from build123d import *

# Parameters (mm, degrees)
SKETCH046_R           = 18.65
SKETCH046_R_2         = 6.05
PAD013_DEPTH          = 2
HOLE001_D             = 3
HOLE001_CSINK_D       = 6.1
HOLE001_CSINK_ANGLE   = 90
POLARPATTERN002_COUNT = 5


with BuildPart() as part:
    # Sketch046 → Pad013 (new body)
    with BuildSketch(Plane.XY.offset(20.5)):
        Circle(SKETCH046_R)
        Circle(SKETCH046_R_2, mode=Mode.SUBTRACT)
    extrude(amount=PAD013_DEPTH)

    # Hole001 (through all)
    with Locations(Plane.XY.offset(22.5)):
        with Locations((10.881279, 7.905712)):
            hole001 = CounterSinkHole(HOLE001_D / 2, HOLE001_CSINK_D / 2, counter_sink_angle=HOLE001_CSINK_ANGLE)

    # PolarPattern002: Hole001 ×5 about axis
    polarpattern002_axis = Axis((0, 0, 22.5), (0, 0, 1))
    for i in range(1, POLARPATTERN002_COUNT):
        add(hole001.rotate(polarpattern002_axis, i * 360 / POLARPATTERN002_COUNT), mode=Mode.SUBTRACT)


solid = part.part
The model under review builds one solid part; all positions refer to its coordinate system, in mm. Give positions to 0.01 mm unless a question says otherwise; leave off trailing zeros. Loops run counter-clockwise (first coordinate to the right, second up) from the corner with the lowest first, then second, coordinate; pieces in that order, holes last. Notation, with made-up numbers: (77, 6) -> (86, 6) arc R18 cw to (86, 29) -> close; hole circle Ø5 at (-11.75, 22.5). An arc over 180 degrees is marked (long way). Answer as a JSON object with one key per item and string values. Group by question number.
Q1. Take a section at D-D (x = 4.5). Write out the cut boundary in (y, z), plus the area to 3 significant figures.
Q2. Wall thickness on line 1 along Y through (x, z) = (0, 21); line 2 along Y through (x, z) = (13, 21.9); line 3 along X through (y, z) = (-2, 21.75): over which ranges is each line inside the solid? List them lowest first.
Q3. Take a section at C-C (z = 22.1). Write out the cut boundary in (x, y).
Q4. Take a section at B-B (x = 0). Write out the cut boundary in (y, z).
Q5. Insertion check: pin 1 (1.8 mm diameter, centred on x = -4.16, y = -12.79, fed in from +Z); pin 2 (4 mm diameter, centred on x = 10.88, y = -7.91, fed in from +Z); pin 3 (1 mm diameter, centred on x = 14, z = 21.5, fed in from +Y). Each pin has a flat end and moves straight along its axis. Give the tip position at first contact, or say it passes through.
Q6. Take a section at A-A (y = 0). Write out the cut boundary in (x, z).
Q7. Draft analysis for pull direction Y (two halves, no side actions). For faces 1 (the cylindrical face through (9.59, -8.67, 20.72)), 2 (the cylindrical face through (-14.8, -11.35, 21.49)), 3 (the flat face through (-4.4, 4.4, 20.5)), state which applies: pulls with the +Y half, pulls with the -Y half, needs draft (parallel to the pull), parting line crosses it, or undercut.
Answer below:
{
 "1": {"outline": "(-18.1, 20.5) -> (-4.04, 20.5) -> (-4.04, 22.5) -> (-18.1, 22.5) -> close; (4.04, 20.5) -> (18.1, 20.5) -> (18.1, 22.5) -> (4.04, 22.5) -> close", "area": "56.2 mm2"},
 "2": {"line 1": "y = -18.65 to -6.05, 6.05 to 18.65", "line 2": "y = -13.37 to -9.14, -6.68 to 6.68, 9.14 to 13.37", "line 3": "x = -18.54 to -14.59, -12.31 to -5.71, 5.71 to 18.54"},
 "3": {"outline": "circle Ø37.3 at (0, 0); hole circle Ø5.3 at (-13.45, 0); hole circle Ø5.3 at (-4.16, -12.79); hole circle Ø5.3 at (-4.16, 12.79); hole circle Ø12.1 at (0, 0); hole circle Ø5.3 at (10.88, -7.91); hole circle Ø5.3 at (10.88, 7.91)"},
 "4": {"outline": "(-18.65, 20.5) -> (-6.05, 20.5) -> (-6.05, 22.5) -> (-18.65, 22.5) -> close; (6.05, 20.5) -> (18.65, 20.5) -> (18.65, 22.5) -> (6.05, 22.5) -> close"},
 "5": {"pin 1": "passes through", "pin 2": "stops at z = 21.45", "pin 3": "stops at y = 12.87"},
 "6": {"outline": "(-18.65, 20.5) -> (-14.95, 20.5) -> (-14.95, 20.95) -> (-16.5, 22.5) -> (-18.65, 22.5) -> close; (-11.95, 20.5) -> (-6.05, 20.5) -> (-6.05, 22.5) -> (-10.4, 22.5) -> (-11.95, 20.95) -> close; (6.05, 20.5) -> (18.65, 20.5) -> (18.65, 22.5) -> (6.05, 22.5) -> close"},
 "7": {"face 1": "undercut", "face 2": "parting line crosses it", "face 3": "needs draft"}
}
